The model under review builds one solid part; all positions refer to its coordinate system, in mm. A direction names the side the tool comes from. Round coordinates to 2 decimals unless told otherwise and drop trailing zeros. Order: outer loops, then holes, each group sorted by start corner. A loop starts at its lowest first (then second) coordinate and runs counter-clockwise, first axis right, second up. Notation, with made-up numbers: (-38.75, -11.5) - (3.25, -11.5) arc R29 cw to (3.25, 24.5) - close; hole circle Ø6 at (68.25, 48). An arc over 180 degrees is marked (long way). One line per question, with ' | ' between items. Start each with the question number.
Item 1: Add section B-B on x = -14. State the section outline as (y, z) points.
Item 2: For L1, parallel to X at y = 12.5, z = -10; L2, parallel to Y at x = 14.5, z = -8.25; L3, parallel to Y at x = 16, z = -8.25, list the stretches that pass through material, from the lowest coordinate up. Write a range as [from, to].
Item 3: Insertion check: pin 1 Ø0.7 at (y, z) = (7, -5) entering from +X; pin 2 Ø6 at (y, z) = (-6.5, -4) entering from +X; pin 3 Ø1.5 at (y, z) = (28, -8.5) entering from -X. Each pin has a flat end and moves straight along its axis. Give the tip position at first contact, or say it passes through.
Item 4: Add section A-A on y = 27. State the section outline as (x, z) points, and give its area (3 significant figures).
Item 5: Draft analysis for pull direction X (two halves, no side actions). For faces 1 (the face through (2.33, -11.6, -6.26)), 2 (the face through (13.1, 19.2, 0)), 3 (the face through (14.112, 13, -6)), state which applies: +X half, -X half, draft (parallel to the pull), parting line (faces both ways), or undercut.
Item 6: Tool access review of faces 4 (the face through (13.1, 19.2, -12.7)), 5 (the face through (4.545, 7.843, -6.261)): name each direction out of +Z, -Z, +X, -X, +Y, -Y from which nothing blocks a thin tool from reaching the whole face with its end or side.
Autodesk Inventor part; units mm, degrees
ref_plane "YZ Plane" through (0, 0, 0) normal (1, 0, 0) x (0, 1, 0)
ref_plane "XZ Plane" through (0, 0, 0) normal (0, 1, 0) x (-1, 0, 0)
ref_plane "XY Plane" through (0, 0, 0) normal (0, 0, 1) x (1, 0, 0)
sketch "Sketch1" plane through (0, 0, 0) normal (0, 0, 1) x (1, 0, 0)
  line L0 (7.8314, 13.1968) -> (7.8314, 20.4485) construction
  line L1 (7.8314, 13.1968) -> (14.1116, 16.8227) construction
  circle A0 centre (7.8314, 13.1968) radius 6.35 construction
  line L2 (7.8314, 13.1968) -> (14.1116, 9.571) construction
  line L3 (7.8314, 13.1968) -> (7.8314, 5.9451) construction
  line L4 (7.8314, 13.1968) -> (1.5513, 9.571) construction
  line L5 (7.8314, 13.1968) -> (1.5513, 16.8227) construction
  line L6 (7.8314, 20.4485) -> (14.1116, 16.8227)
  line L7 (14.1116, 16.8227) -> (14.1116, 9.571)
  line L8 (7.8314, 5.9451) -> (14.1116, 9.571)
  line L9 (7.8314, 5.9451) -> (1.5513, 9.571)
  line L10 (1.5513, 9.571) -> (1.5513, 16.8227)
  line L11 (1.5513, 16.8227) -> (7.8314, 20.4485)
  circle A1 centre (7.8314, 13.1968) radius 25.4
  circle A2 centre (7.8314, 20.4485) radius 2.3813
  circle A3 centre (14.1116, 16.8227) radius 2.3813
  circle A4 centre (14.1116, 9.571) radius 2.3813
  circle A5 centre (7.8314, 5.9451) radius 2.3813
  circle A6 centre (1.5513, 9.571) radius 2.3813
  circle A7 centre (1.5513, 16.8227) radius 2.3813
  line L12 (5.4502, 19.9903) -> (10.2127, 19.9903)
  line L13 (10.2127, 19.9903) -> (10.2127, 19.0737)
  line L14 (10.2127, 19.0737) -> (5.4502, 19.0737)
  line L15 (5.4502, 19.0737) -> (5.4502, 19.9903)
  line L16 (11.9019, 8.2952) -> (12.6147, 7.719)
  line L17 (12.6147, 7.719) -> (15.6085, 11.4229)
  line L18 (15.6085, 11.4229) -> (14.8957, 11.9991)
  line L19 (14.8957, 11.9991) -> (11.9019, 8.2952)
  line L20 (5.4502, 7.3199) -> (5.4502, 6.4034)
  line L21 (5.4502, 6.4034) -> (10.2127, 6.4034)
  line L22 (10.2127, 6.4034) -> (10.2127, 7.3199)
  line L23 (10.2127, 7.3199) -> (5.4502, 7.3199)
  line L24 (1.5513, 12.1225) -> (0.6959, 11.7933)
  line L25 (0.6959, 11.7933) -> (2.4066, 7.3487)
  line L26 (2.4066, 7.3487) -> (3.262, 7.6779)
  line L27 (3.262, 7.6779) -> (1.5513, 12.1225)
  line L28 (3.761, 18.0984) -> (3.0482, 18.6746)
  line L29 (3.0482, 18.6746) -> (0.0544, 14.9707)
  line L30 (0.0544, 14.9707) -> (0.7672, 14.3946)
  line L31 (0.7672, 14.3946) -> (3.761, 18.0984)
  line L32 (14.1116, 14.073) -> (14.9053, 14.5313)
  line L33 (14.9053, 14.5313) -> (12.5241, 18.6558)
  line L34 (12.5241, 18.6558) -> (11.7303, 18.1975)
  line L35 (11.7303, 18.1975) -> (14.1116, 14.073)
  circle A8 centre (7.8314, 13.1968) radius 4.0132 construction
  dimension "d9" = 4.7625
  dimension "d11" = 4.7625
  dimension "d0" = 7.2517
  dimension "d1" = 12.7
  dimension "d2" = 60
  dimension "d3" = 60
  dimension "d4" = 60
  dimension "d5" = 60
  dimension "d6" = 60
  dimension "d7" = 4.7625
  dimension "d8" = 4.7625
  dimension "d10" = 4.7625
  dimension "d12" = 4.7625
  dimension "d13" = 50.8
  dimension "d14" = 0.9165
  dimension "d16" = 0.9165
  dimension "d17" = 0.9165
  dimension "d18" = 0.9165
  dimension "d19" = 0.9165
  dimension "d20" = 0.9165
  dimension "d24" = 2.3368
extrude "Extrusion1" add sketch "Sketch1" against normal blind 12.7
equation "\"d9\" = d7"
equation "\"d11\" = d7"
equation "\"d8\" = d7"
equation "\"d10\" = d7"
equation "\"d12\" = d7"
properties part number "augmented gear v2"
Determined:
1) outline: (0.21, -12.7) - (26.18, -12.7) - (26.18, 0) - (0.21, 0) - close
2) L1: [-17.56, 1.55], [14.11, 33.22] | L2: [-11.31, 7.22], [11.92, 14.3], [19.17, 37.71] | L3: [-10.85, 8.12], [11.02, 15.37], [18.27, 37.25]
3) pin 1: x = 32.55 | pin 2: x = 26.97 | pin 3: x = -13.33
4) outline: (-13.49, -12.7) - (29.15, -12.7) - (29.15, 0) - (-13.49, 0) - close | area: 542 mm2
5) face 1: parting line | face 2: draft | face 3: undercut
6) face 4: -Z, +X, -X, +Y, -Y | face 5: +Z, -Z
